Source: CAD feature listing. Evaluate the final solid. Frame: model axes, mm. A direction names the side the tool comes from. Give positions to 0.01 mm unless a question says otherwise; leave off trailing zeros. Order: outer loops, then holes, each group sorted by start corner. A loop starts at its lowest first (then second) coordinate and runs counter-clockwise, first axis right, second up.
```python
from build123d import *

# Parameters (mm, degrees)
SKETCH_1_W          = 35
SKETCH_1_H          = 35
EXTRUDE_1_DEPTH     = 5.2
SKETCH_2_R          = 18
EXTRUDE_2_DEPTH     = 32.8
SKETCH_3_R          = 11
EXTRUDE_3_DEPTH     = 2
SKETCH_4_R          = 4
EXTRUDE_4_DEPTH     = 18
SKETCH_5_W          = 10.54681648
SKETCH_5_H          = 7.766292135
CUT_EXTRUDE_1_DEPTH = 15
CHAMFER_1_SIZE      = 2
SKETCH_6_R          = 1.5
CUT_EXTRUDE_2_DEPTH = 6
SKETCH_7_R          = 1.5
CUT_EXTRUDE_3_DEPTH = 6


with BuildPart() as part:
    # 草图1 → 凸台-拉伸1 (new body)
    with BuildSketch(Plane(origin=(0, 0, 0), x_dir=(1, 0, 0), z_dir=(0, 1, 0))):
        Rectangle(SKETCH_1_W, SKETCH_1_H)
    extrude(amount=EXTRUDE_1_DEPTH)

    # 草图2 → 凸台-拉伸2 (add)
    with BuildSketch(Plane(origin=(0, 5.2, 0), x_dir=(1, 0, 0), z_dir=(0, 1, 0))):
        with Locations(Location((0, 0, 0), (0, 0, 76.463797263))):
            Circle(SKETCH_2_R)
    extrude(amount=EXTRUDE_2_DEPTH)

    # 草图3 → 凸台-拉伸3 (add)
    with BuildSketch(Plane(origin=(0, 38, 0), x_dir=(1, 0, 0), z_dir=(0, 1, 0))):
        with Locations(Location((0, 0, 0), (0, 0, 270))):
            Circle(SKETCH_3_R)
    extrude(amount=EXTRUDE_3_DEPTH)

    # 草图4 → 凸台-拉伸4 (add)
    with BuildSketch(Plane(origin=(0, 40, 0), x_dir=(1, 0, 0), z_dir=(0, 1, 0))):
        with Locations(Location((0, 0, 0), (0, 0, 270))):
            Circle(SKETCH_4_R)
    extrude(amount=EXTRUDE_4_DEPTH)

    # 草图5 → 切除-拉伸1 (cut)
    with BuildSketch(Plane(origin=(0, 58, 0), x_dir=(1, 0, 0), z_dir=(0, 1, 0))):
        with Locations((0, 6.883146068)):
            Rectangle(SKETCH_5_W, SKETCH_5_H)
    extrude(amount=-CUT_EXTRUDE_1_DEPTH, mode=Mode.SUBTRACT)

    # 倒角1
    chamfer_1_edges = [part.edges().sort_by_distance(p)[0] for p in [
        (17.5, 2.6, 17.5),
        (-17.5, 2.6, 17.5),
        (-17.5, 2.6, -17.5),
        (17.5, 2.6, -17.5),
    ]]
    chamfer(chamfer_1_edges, length=CHAMFER_1_SIZE)

    # 草图6 → 切除-拉伸2 (cut)
    with BuildSketch(Plane(origin=(0, 38, 0), x_dir=(1, 0, 0), z_dir=(0, 1, 0))):
        with Locations(Location((0, 14, 0), (0, 0, 270))):
            Circle(SKETCH_6_R)
        with Locations(Location((14, 0, 0), (0, 0, 270))):
            Circle(SKETCH_6_R)
        with Locations(Location((0, -14, 0), (0, 0, 270))):
            Circle(SKETCH_6_R)
        with Locations(Location((-14, 0, 0), (0, 0, 270))):
            Circle(SKETCH_6_R)
    extrude(amount=-CUT_EXTRUDE_2_DEPTH, mode=Mode.SUBTRACT)

    # 草图7 → 切除-拉伸3 (cut)
    with BuildSketch(Plane(origin=(0, 38, 0), x_dir=(1, 0, 0), z_dir=(0, 1, 0))):
        with Locations(Location((-9.899494937, 9.899494937, 0), (0, 0, 270))):
            Circle(SKETCH_7_R)
        with Locations(Location((9.899494937, 9.899494937, 0), (0, 0, 270))):
            Circle(SKETCH_7_R)
        with Locations(Location((9.899494937, -9.899494937, 0), (0, 0, 270))):
            Circle(SKETCH_7_R)
        with Locations(Location((-9.899494937, -9.899494937, 0), (0, 0, 270))):
            Circle(SKETCH_7_R)
    extrude(amount=-CUT_EXTRUDE_3_DEPTH, mode=Mode.SUBTRACT)


solid = part.part
```
1) Reachability of faces 1 (the flat face through (17.5, 3, 0)), 2 (the cylindrical face through (-10.74, 38.99, -2.38)), 3 (the flat face through (0, 3, -17.5)) from +Z, -Z, +X, -X, +Y, -Y: full face, straight path, thin tool, end or side. Return the list, or none.
Report:
face 1: +Z, -Z, +X, -Y
face 2: +Y
face 3: -Z, +X, -X, -Y
2) Section query A-A, the plane x = 0. Return the cut outline in (y, z), and give its area (3 significant figures).
Report:
outline: (0, -17.5) - (5.2, -17.5) - (5.2, -18) - (38, -18) - (38, -15.5) - (32, -15.5) - (32, -12.5) - (38, -12.5) - (38, -11) - (40, -11) - (40, -4) - (43, -4) - (43, -3) - (58, -3) - (58, 4) - (40, 4) - (40, 11) - (38, 11) - (38, 12.5) - (32, 12.5) - (32, 15.5) - (38, 15.5) - (38, 18) - (5.2, 18) - (5.2, 17.5) - (0, 17.5) - close
area: 1,500 mm2
3) Section query B-B, the plane z = 0. Return the cut outline in (x, y), and give its area (3 significant figures).
Report:
outline: (-18, 5.2) - (-17.5, 5.2) - (-17.5, 0) - (17.5, 0) - (17.5, 5.2) - (18, 5.2) - (18, 38) - (15.5, 38) - (15.5, 32) - (12.5, 32) - (12.5, 38) - (11, 38) - (11, 40) - (4, 40) - (4, 58) - (-4, 58) - (-4, 40) - (-11, 40) - (-11, 38) - (-12.5, 38) - (-12.5, 32) - (-15.5, 32) - (-15.5, 38) - (-18, 38) - close
area: 1,510 mm2
4) Section query D-D, the plane y = 16. Return the cut outline in (x, z).
Report:
outline: circle Ø36 at (0, 0)
5) Material intervals for L1, parallel to X at y = 35.55, z = 0; L2, parallel to Z at x = 13.5, y = 4.5; L3, parallel to Y at x = -13.5, z = -0.5, sorted ascending.
Report:
L1: x = -18 to -15.5, -12.5 to 12.5, 15.5 to 18
L2: z = -17.5 to 17.5
L3: y = 0 to 32
6) Pin query (flat end, axial travel): pin 1 (10 mm diameter, centred on y = 40.5, z = 1.5, fed in from +X); pin 2 (12 mm diameter, centred on y = 31, z = 13.5, fed in from +X); pin 3 (0.9 mm diameter, centred on x = -10, z = 9.5, fed in from +Y); pin 4 (6 mm diameter, centred on x = 0.5, y = 47.5, fed in from -Z). Return the tip coordinate at first contact, or that it passes through.
Report:
pin 1: stops at x = 18
pin 2: stops at x = 16.36
pin 3: stops at y = 32
pin 4: stops at z = -3
7) Draft query along Z for faces 4 (the cylindrical face through (0.07, 35.04, -15.5)), 5 (the flat face through (-16, 3, 17)), 6 (the flat face through (0, 0, 0)). Return one class per face: +Z half, -Z half, draft (parallel to the pull), parting line (faces both ways), or undercut.
Report:
face 4: undercut
face 5: +Z half
face 6: draft
8) Section query C-C, the plane y = 36.5. Count the separate pieces of the cut face and the enclosed holes in it, and give its area (3 significant figures).
Report:
separate pieces: 1
enclosed holes: 8
area: 961 mm2
